from build123d import *


with BuildPart() as f1:
    # F0 (on Right) → F1 (revolve)
    with BuildSketch(Plane.YZ):
        with BuildLine():
            Line((8, 38.75), (0, 38.75))
            Line((0, 38.75), (0, 39.75))
            ThreePointArc((0, 39.75), (-0.87868, 41.87132), (-3, 42.75))
            Line((-3, 42.75), (-7, 42.75))
            ThreePointArc((-7, 42.75), (-8.65, 41.669375), (-10.3, 42.75))
            Line((-10.3, 42.75), (-14.3, 42.75))
            ThreePointArc((-14.3, 42.75), (-15.893266, 42.291949), (-17, 41.05767))
            Line((-17, 41.05767), (-17, 12))
            Line((-17, 12), (-10, 12))
            Line((-10, 12), (-10, 5.5))
            Line((-10, 5.5), (8, 5.5))
            Line((8, 5.5), (8, 38.75))
        make_face()
    revolve(axis=Axis((0, 0.134684, 0), (0, 1, 0)))


solid = f1.part
The listing builds one solid part. Answer for the finished solid, in the listing's coordinates (mm). A direction names the side the tool comes from. Coordinates: 2 decimals unless noted, no trailing zeros. Loops run counter-clockwise (first coordinate to the right, second up) from the corner with the lowest first, then second, coordinate; pieces in that order, holes last. Notation, with made-up numbers: (-23, 50) -> (-10, 50) arc R7 cw to (-10, 59) -> close; hole circle Ø4 at (59, 53). An arc over 180 degrees is marked (long way). Write item = value, one per line. Start each with the question number.
1) A cutting plane is placed at D-D (y = 6). Give the vertices of the cut face in (x, z).
2) A cutting plane is placed at A-A (x = 0). Give the vertices of the cut face in (y, z), then the cut area to 3 significant figures.
3) Given pin 1 Ø3 at (y, z) = (-3, -24) entering from -X; pin 2 Ø6.5 at (x, z) = (0, 0) entering from -Y; pin 3 Ø4 at (x, y) = (-29.5, -9.5) entering from +Z; pin 4 Ø19 at (x, z) = (-2, 0.5) entering from -Y, each flat-ended and moving along its own axis, determine where each tip first touches the part or whether it passes through.
4) Straight lines are drawn through the part: line 1 (X direction, y = 2.5, z = 0); line 2 (X direction, y = -6, z = 0); line 3 (Z direction, x = -6, y = -15.5). For each, find the intervals that lie inside material, in ascending order. Write a range as from..to.
5) The mould has two halves that part along X. Classify faces 4 (the face through (-5.37, -0.87, -1.19)), 5 (the face through (12.841, -5.028, 40.776)), 6 (the face through (-8, 8, 1)): released by +X, released by -X, zero draft, split by the parting line, or undercut.
6) A cutting plane is placed at C-C (y = -4.5). Give the vertices of the cut face in (x, z).
7) A tool of negligible diameter and unlimited length cuts with its end or side. For faces 1 (the face through (-2.5, -10, 5.2)), 2 (the face through (12.841, -12.328, 40.776)), 3 (the face through (-38, 0, -9)), from which of +Z, -Z, +X, -X, +Y, -Y can it reach the whole face along a straight path? Write none if from no direction.
8) A cutting plane is placed at B-B (z = 0). Give the vertices of the cut face in (x, y).
Responses:
q1.outline = circle Ø77.5 at (0, 0); hole circle Ø11 at (0, 0)
q2.outline = (-17, -41.06) arc R3 ccw to (-14.3, -42.75) -> (-10.3, -42.75) arc R1.8 cw to (-7, -42.75) -> (-3, -42.75) arc R3 ccw to (0, -39.75) -> (0, -38.75) -> (8, -38.75) -> (8, -5.5) -> (-10, -5.5) -> (-10, -12) -> (-17, -12) -> close; (-17, 12) -> (-10, 12) -> (-10, 5.5) -> (8, 5.5) -> (8, 38.75) -> (0, 38.75) -> (0, 39.75) arc R3 ccw to (-3, 42.75) -> (-7, 42.75) arc R1.8 cw to (-10.3, 42.75) -> (-14.3, 42.75) arc R3 ccw to (-17, 41.06) -> close
q2.area = 1,700 mm²
q3.pin_1 = -36.35
q3.pin_2 = through
q3.pin_3 = 32.59
q3.pin_4 = -10
q4.line_1 = -38.75..-5.5, 5.5..38.75
q4.line_2 = -42.75..-5.5, 5.5..42.75
q4.line_3 = -42.07..-10.39, 10.39..42.07
q5.face_4 = undercut
q5.face_5 = split by the parting line
q5.face_6 = zero draft
q6.outline = circle Ø85.5 at (0, 0); hole circle Ø11 at (0, 0)
q7.face_1 = -Y
q7.face_2 = +Y, -Y
q7.face_3 = +Y
q8.outline = (-42.75, -14.3) arc R3 ccw to (-41.06, -17) -> (-12, -17) -> (-12, -10) -> (-5.5, -10) -> (-5.5, 8) -> (-38.75, 8) -> (-38.75, 0) -> (-39.75, 0) arc R3 ccw to (-42.75, -3) -> (-42.75, -7) arc R1.8 cw to (-42.75, -10.3) -> close; (5.5, -10) -> (12, -10) -> (12, -17) -> (41.06, -17) arc R3 ccw to (42.75, -14.3) -> (42.75, -10.3) arc R1.8 cw to (42.75, -7) -> (42.75, -3) arc R3 ccw to (39.75, 0) -> (38.75, 0) -> (38.75, 8) -> (5.5, 8) -> close
